```python
from build123d import *

# Parameters (mm, degrees)
BOSS_EXTRUDE1_DEPTH = 76.2
FILLET1_R           = 3.175
SKETCH4_R           = 2.778125
CUT_EXTRUDE1_DEPTH  = 6.35


with BuildPart() as part:
    # Sketch1 → Boss-Extrude1 (new body)
    with BuildSketch(Plane.XY):
        Polygon((0, 0), (14.2875, 0), (14.2875, 38.1), (90.4875, 38.1), (90.4875, 0), (104.775, 0), (104.775, 2.38125), (95.25, 2.38125), (95.25, 41.275), (9.525, 41.275), (9.525, 2.38125), (0, 2.38125), align=None)
    extrude(amount=BOSS_EXTRUDE1_DEPTH)

    # Fillet1
    fillet1_edges = [part.edges().sort_by_distance(p)[0] for p in [
        (9.525, 2.38125, 38.1),
        (9.525, 41.275, 38.1),
        (95.25, 41.275, 38.1),
        (95.25, 2.38125, 38.1),
        (90.4875, 38.1, 38.1),
        (14.2875, 38.1, 38.1),
    ]]
    fillet(fillet1_edges, radius=FILLET1_R)

    # Sketch4 → Cut-Extrude1 (cut, symmetric)
    with BuildSketch(Plane(origin=(0, 2.38125, 0), x_dir=(1, 0, 0), z_dir=(0, 1, 0))):
        with Locations(Location((100.0125, -12.7, 0), (0, 0, 235.150095421))):
            Circle(SKETCH4_R)
        with Locations(Location((100.0125, -63.5, 0), (0, 0, 235.150095421))):
            Circle(SKETCH4_R)
        with Locations(Location((4.7625, -63.5, 0), (0, 0, 270))):
            Circle(SKETCH4_R)
        with Locations(Location((4.7625, -12.7, 0), (0, 0, 270))):
            Circle(SKETCH4_R)
    extrude(amount=CUT_EXTRUDE1_DEPTH, both=True, mode=Mode.SUBTRACT)


solid = part.part
```
Read the model definition and answer for the solid it produces. Units are mm, in the model's axes. A direction names the side the tool comes from. Coordinates: 2 decimals unless noted, no trailing zeros. Write each loop counter-clockwise with the first axis right and the second up, starting at its lowest first coordinate (ties: lowest second). Pieces come first, ordered by that corner, then holes. Notation, with made-up numbers: (32.25, -14.75) - (58.25, -14.75) arc R34 cw to (58.25, 23.25) - close; hole circle Ø5 at (56.25, 50.5). An arc over 180 degrees is marked (long way). Answer as a JSON object with one key per item and string values. Group by question number.
1. A cutting plane is placed at A-A (z = 63.5). Give the number of separate pieces and of enclosed holes in the cut face, plus the area to 3 significant figures.
2. Each of these flat-tipped pins is pushed along its axis until it touches: P1, Ø8, axis at y = 14.5, z = 17.5, coming from the -X side (3 decimals); P2, Ø17.5, axis at y = 23, z = 56, coming from the +X side; P3, Ø1.9, axis at x = 101, z = 42, coming from the +Y side. Where does it stop, or does it pass through?
3. The mould has two halves that part along Z. Classify faces 1 (the cylindrical face through (97.257, 1.325, 12.344)), 2 (the flat face through (0, 1, 38)), 3 (the flat face through (60, 39, 76.2)): +Z half, -Z half, draft (parallel to the pull), parting line (faces both ways), or undercut.
4. Which of the six approach directions +Z, -Z, +X, -X, +Y, -Y give full straight-line access (tool end or side, diameter ignored) to faces 4 (the flat face through (14.288, 17, 38)), 5 (the flat face through (3, 2.381, 38)), 6 (the flat face through (102, 2.381, 38))?
5. A cutting plane is placed at D-D (x = 56). Determine the outline of the cut face in (y, z) (3 decimals), plus the area to 3 significant figures.
6. Consider L1, parallel to X at y = 1.1, z = 63.5 (1 decimal); L2, parallel to X at y = 2, z = 31.5 (1 decimal); L3, parallel to X at y = 1, z = 12 (1 decimal). Determine where each line is inside the solid, lowest interval first. Write a range as [from, to].
Worked out:
{
 "1": {"separate pieces": "3", "enclosed holes": "0", "area": "658 mm²"},
 "2": {"P1": "stops at x = 9.525", "P2": "stops at x = 95.25", "P3": "stops at y = 2.38"},
 "3": {"face 1": "undercut", "face 2": "draft", "face 3": "+Z half"},
 "4": {"face 4": "+Z, -Z, -Y", "face 5": "+Z, -Z, -X, +Y", "face 6": "+Z, -Z, +X, +Y"},
 "5": {"outline": "(38.1, 0) - (41.275, 0) - (41.275, 76.2) - (38.1, 76.2) - close", "area": "242 mm²"},
 "6": {"L1": "x = [0, 2], [7.5, 14.3], [90.5, 97.2], [102.8, 104.8]", "L2": "x = [0, 14.3], [90.5, 104.8]", "L3": "x = [0, 2.1], [7.5, 14.3], [90.5, 97.3], [102.7, 104.8]"}
}
